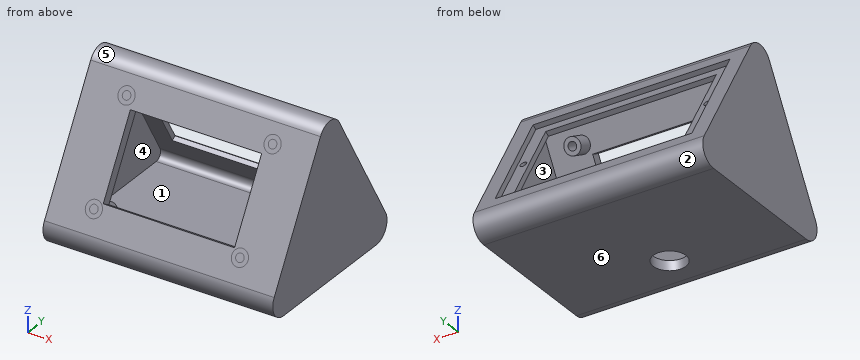
```python
from build123d import *

# Parameters (mm, degrees)
F1_DEPTH  = 35
F2_DEPTH  = 32
F3_R      = 5
F4_R      = 2
F5_W      = 40
F5_H      = 25
F6_DEPTH  = 3
F5_R      = 2.5
F5_R_2    = 1.25
F7_DEPTH  = 8
F8_W      = 52
F8_H      = 29
F9_DEPTH  = 3
F8_W_2    = 60
F8_H_2    = 35
F10_DEPTH = 1.5
F11_R     = 5
F12_DEPTH = 3
F13_D     = 2
F13_DEPTH = 3
F13_TIP   = 0.600860619


with BuildPart() as f1:
    # F0 (on Right) → F1 (new body, symmetric)
    with BuildSketch(Plane.YZ):
        Polygon((-60, 0), (0, 0), (-30, 51.9615242271), align=None)
        Polygon((-5.1961524227, 3), (-54.8038475773, 3), (-30, 45.9615242271), align=None, mode=Mode.SUBTRACT)
        Polygon((-30, 45.9615242271), (-54.8038475773, 3), (-5.1961524227, 3), align=None)
    extrude(amount=F1_DEPTH, both=True)

    # F0 (on Right) → F2 (cut, symmetric)
    with BuildSketch(Plane.YZ):
        Polygon((-30, 45.9615242271), (-54.8038475773, 3), (-5.1961524227, 3), align=None)
    extrude(amount=F2_DEPTH, both=True, mode=Mode.SUBTRACT)

    # F3
    f3_edges = [f1.edges().sort_by_distance(p)[0] for p in [
        (0, -30, 51.961524),
        (0, -60, 0),
        (0, 0, 0),
    ]]
    fillet(f3_edges, radius=F3_R)

    # F4
    f4_edges = [f1.edges().sort_by_distance(p)[0] for p in [
        (0, -30, 45.961524),
        (0, -5.196152, 3),
        (0, -54.803848, 3),
    ]]
    fillet(f4_edges, radius=F4_R)

    # F5 (on face) → F6 (cut)
    with BuildSketch(Plane(origin=(0, -45, 25.9807621135), x_dir=(1, 0, 0), z_dir=(0, -0.8660254038, 0.5))):
        with Locations((0, -0.0002540378)):
            Rectangle(F5_W, F5_H)
    extrude(amount=-F6_DEPTH, mode=Mode.SUBTRACT)

    # F5 (on face) → F7 (join)
    with BuildSketch(Plane(origin=(0, -45, 25.9807621135), x_dir=(1, 0, 0), z_dir=(0, -0.8660254038, 0.5))):
        with Locations((-22.1997145563, 15.6450960785)):
            Circle(F5_R)
        with Locations((-22.1997145563, 15.6450960785)):
            Circle(F5_R_2, mode=Mode.SUBTRACT)
        with Locations((22.287291775, 15.6450960785)):
            Circle(F5_R)
        with Locations((22.287291775, 15.6450960785)):
            Circle(F5_R_2, mode=Mode.SUBTRACT)
        with Locations((22.287291775, -14.4981121665)):
            Circle(F5_R)
        with Locations((22.287291775, -14.4981121665)):
            Circle(F5_R_2, mode=Mode.SUBTRACT)
        with Locations((-22.1997145563, -14.4981121665)):
            Circle(F5_R)
        with Locations((-22.1997145563, -14.4981121665)):
            Circle(F5_R_2, mode=Mode.SUBTRACT)
    extrude(amount=-F7_DEPTH)

    # F8 (on face) → F9 (cut)
    with BuildSketch(Plane(origin=(0, 0, 0), x_dir=(-1, 0, 0), z_dir=(0, 0.8660254038, 0.5))):
        with Locations((0, 30.0002540378)):
            Rectangle(F8_W, F8_H)
    extrude(amount=-F9_DEPTH, mode=Mode.SUBTRACT)

    # F8 (on face) → F10 (cut)
    with BuildSketch(Plane(origin=(0, 0, 0), x_dir=(-1, 0, 0), z_dir=(0, 0.8660254038, 0.5))):
        with Locations((0, 30.0002540378)):
            Rectangle(F8_W_2, F8_H_2)
        with Locations((0, 30.0002540378)):
            Rectangle(F8_W, F8_H, mode=Mode.SUBTRACT)
    extrude(amount=-F10_DEPTH, mode=Mode.SUBTRACT)

    # F11 (on face) → F12 (cut, through all)
    with BuildSketch(Plane(origin=(0, 0, 0), x_dir=(1, 0, 0), z_dir=(0, 0, -1))):
        with Locations((0, 41.3397459622)):
            Circle(F11_R)
    extrude(amount=-F12_DEPTH, mode=Mode.SUBTRACT)

    # F13
    with Locations(Plane(origin=(0, 0, 0), x_dir=(-1, 0, 0), z_dir=(0, 0.8660254038, 0.5))):
        with Locations((-28, 30.0002540378), (28, 30.0002540378)):
            Hole(F13_D / 2, depth=F13_DEPTH)
            with Locations((0, 0, -(F13_DEPTH + F13_TIP / 2))):  # 118° drill point
                Cone(0, F13_D / 2, F13_TIP, mode=Mode.SUBTRACT)


solid = f1.part
```
Can you work these out from the model? Positions are in its coordinate system, mm. Face numbers are marked on the shaded views. A direction names the side the tool comes from. Round coordinates to 2 decimals unless told otherwise and drop trailing zeros. Loops run counter-clockwise (first coordinate to the right, second up) from the corner with the lowest first, then second, coordinate; pieces in that order, holes last. Notation, with made-up numbers: M 69.5,82 L 128.5,82 A7 ccw 128.5,90 Z; hole C 13,-37.75 d5. An arc over 180 degrees is marked long. Write item = value, one per line. Start each with the question number.
(1) Suppose I cut it at B-B on x = 0. Write out the boundary of the cut face in (y, z), plus the area to 3 significant figures.
(2) I need wall thicknesses on line 1 along X through (y, z) = (-30.5, 28); line 2 along Z through (x, y) = (1, -51.5); line 3 along Y through (x, z) = (-30.5, 29.5). Which ranges of each line are inside material? Lowest first, please.
(3) I'm going to push flat-ended pins straight in: P1, Ø8, axis at x = 20, z = 38.5, coming from the -Y side; P2, Ø3, axis at y = -45.5, z = 27.5, coming from the -X side; P3, Ø6, axis at x = 0, y = -41.34, coming from the -Z side; P4, Ø3, axis at x = -18.5, y = -21, coming from the +Z side. Where does each tip first touch, or does it pass through?
(4) Suppose I cut it at C-C on x = 31. Write out the boundary of the cut face in (y, z).
(5) Suppose I cut it at D-D on y = -33. Give the number of separate pieces and of enclosed holes in the cut face, plus the area to 3 significant figures.
(6) Suppose I cut it at A-A on x = -18.5. Write out the boundary of the cut face in (y, z).
(7) Which directions (+Z, -Z, +X, -X, +Y, -Y) give clear straight access to the entire face, cutting with the end or side of a thin tool? Please do the marked faces 1 and 2.
(8) If we mould it in two halves opening along Z, with no side actions, what happens to the marked faces 3, 4, 5 and 6? For each: released by +Z, released by -Z, zero draft, split by the parting line, or undercut.
Answer block:
q1.outline = M -55.67,7.5 A5 ccw -51.34,0 L -46.34,0 L -46.34,3 L -51.34,3 A2 cw -53.07,6 L -48.65,13.66 L -51.25,15.16 Z; M -38.75,36.81 L -36.15,35.31 L -31.73,42.96 A2 cw -28.27,42.96 L -24.85,37.04 L -23.55,37.79 L -25.05,40.39 L -23.75,41.14 L -25.67,44.46 A5 ccw -34.33,44.46 Z; M -36.34,0 L -8.66,0 A5 ccw -4.33,7.5 L -6.25,10.83 L -7.55,10.08 L -9.05,12.67 L -10.35,11.92 L -6.93,6 A2 cw -8.66,3 L -36.34,3 Z
q1.area = 249 mm²
q2.line_1 = -35 to -32, 32 to 35
q2.line_2 = 0 to 3.01, 8.72 to 14.72
q2.line_3 = -42.97 to -39.5, -20.5 to -17.03
q3.P1 = -40.08
q3.P2 = -35
q3.P3 = 36.57
q3.P4 = 3
q4.outline = M -55.67,7.5 A5 ccw -51.34,0 L -8.66,0 A5 ccw -4.33,7.5 L -25.67,44.46 A5 ccw -34.33,44.46 Z; hole M -53.07,6 A2 ccw -51.34,3 L -8.66,3 A2 ccw -6.93,6 L -28.27,42.96 A2 ccw -31.73,42.96 Z
q5.separate_pieces = 3
q5.enclosed_holes = 3
q5.area = 834 mm²
q6.outline = M -55.67,7.5 A5 ccw -51.34,0 L -8.66,0 A5 ccw -4.33,7.5 L -6.25,10.83 L -7.55,10.08 L -9.05,12.67 L -10.35,11.92 L -6.93,6 A2 cw -8.66,3 L -51.34,3 A2 cw -53.07,6 L -48.65,13.66 L -51.25,15.16 Z; M -38.75,36.81 L -36.15,35.31 L -31.73,42.96 A2 cw -28.27,42.96 L -24.85,37.04 L -23.55,37.79 L -25.05,40.39 L -23.75,41.14 L -25.67,44.46 A5 ccw -34.33,44.46 Z
q7.face_1 = none
q7.face_2 = +X, -X, +Y
q8.face_3 = undercut
q8.face_4 = undercut
q8.face_5 = released by +Z
q8.face_6 = released by -Z
